Design review of the part built by this model. Coordinates are the model's own, in mm. A direction names the side the tool comes from. Give positions to 0.01 mm unless a question says otherwise; leave off trailing zeros. Loops run counter-clockwise (first coordinate to the right, second up) from the corner with the lowest first, then second, coordinate; pieces in that order, holes last. Notation, with made-up numbers: (17.5, 12.25) -> (21.5, 12.25) arc R17 cw to (21.5, 38.25) -> close; hole circle Ø10 at (87.5, 33). An arc over 180 degrees is marked (long way). Use CSV: the item, a comma, the result in double quotes. Start each with the question number.
Item 1: Clearance check with flat-ended pins moving along their axes: pin 1 (3.5 mm diameter, centred on x = 17.68, y = 17.68, fed in from +Z); pin 2 (3 mm diameter, centred on x = 19.5, y = -1.5, fed in from +Z); pin 3 (10 mm diameter, centred on x = -9.5, z = -25.5, fed in from -Y). State where each tip first meets the part, or that it passes through.
Item 2: Wall thickness on line 1 along Y through (x, z) = (0, -17); line 2 along Y through (x, z) = (0, -25); line 3 along Z through (x, y) = (-35.5, 26.5): over which ranges is each line inside the solid? List them lowest first. Write a range as from..to.
Item 3: We need section D-D (x = 31). State the section outline as (y, z) points, plus the area to 3 significant figures.
Item 4: We need section A-A (x = 0). State the section outline as (y, z) points, plus the area to 3 significant figures.
Item 5: We need section C-C (y = 30). State the section outline as (x, z) points, plus the area to 3 significant figures.
Item 6: The part is to be moulded in two halves that separate along X. For faces 1 (the face through (-20, 0, -20)), 2 (the face through (50.934, 16.04, -18.98)), 3 (the face through (-1, -11, -38.5)), say which applies: +X half, -X half, draft (parallel to the pull), parting line (faces both ways), or undercut.
Item 7: For faces 4 (the face through (-1.73, -7.81, -17.97)), 5 (the face through (20, 0, -20)), 6 (the face through (0.33, -27.52, -28.64)), list the 3-axis set-ups (+Z, -Z, +X, -X, +Y, -Y) from which the entire face can be reached by the end or side of a thin tool; tool diameter is ignored.
from build123d import *

# Parameters (mm, degrees)
SKETCH3_R           = 53.4
BOSS_EXTRUDE1_DEPTH = 38.5
SKETCH4_R           = 8
CUT_EXTRUDE1_DEPTH  = 85.766561804
SKETCH5_R           = 2
CUT_EXTRUDE2_DEPTH  = 20
BOSS_EXTRUDE3_START = 2
SKETCH6_R           = 16
SKETCH6_R_2         = 8
BOSS_EXTRUDE3_DEPTH = 2
SKETCH7_R           = 2.1
CUT_EXTRUDE3_DEPTH  = 20
SKETCH8_R           = 2.5
CUT_EXTRUDE4_DEPTH  = 20


with BuildPart() as part:
    # Sketch3 → Boss-Extrude1 (new body)
    with BuildSketch(Plane.XY):
        Circle(SKETCH3_R)
    extrude(amount=-BOSS_EXTRUDE1_DEPTH)

    # Sketch4 → Cut-Extrude1 (cut, through all)
    with BuildSketch(Plane.XY):
        Circle(SKETCH4_R)
    extrude(amount=-CUT_EXTRUDE1_DEPTH, mode=Mode.SUBTRACT)

    # Sketch5 → Cut-Extrude2 (cut)
    with BuildSketch(Plane.XY):
        with Locations((-17.67766953, 17.67766953)):
            Circle(SKETCH5_R)
        with Locations((17.67766953, 17.67766953)):
            Circle(SKETCH5_R)
        with Locations((-17.67766953, -17.67766953)):
            Circle(SKETCH5_R)
        with Locations((17.67766953, -17.67766953)):
            Circle(SKETCH5_R)
    extrude(amount=-CUT_EXTRUDE2_DEPTH, mode=Mode.SUBTRACT)

    # Sketch6 → Boss-Extrude3 (add)
    with BuildSketch(Plane.XY.offset(BOSS_EXTRUDE3_START)):
        Circle(SKETCH6_R)
        Circle(SKETCH6_R_2, mode=Mode.SUBTRACT)
    extrude(amount=-BOSS_EXTRUDE3_DEPTH)

    # Sketch7 → Cut-Extrude3 (cut)
    with BuildSketch(Plane.XY):
        with Locations((0, 20)):
            Circle(SKETCH7_R)
        with Locations((20, 0)):
            Circle(SKETCH7_R)
        with Locations((-20, 0)):
            Circle(SKETCH7_R)
        with Locations((0, -20)):
            Circle(SKETCH7_R)
    extrude(amount=-CUT_EXTRUDE3_DEPTH, mode=Mode.SUBTRACT)

    # Sketch8 → Cut-Extrude4 (cut)
    with BuildSketch(Plane(origin=(0, 0, -38.5), x_dir=(-1, 0, 0), z_dir=(0, 0, -1))):
        with Locations((0, 30)):
            Circle(SKETCH8_R)
        with Locations((30, 0)):
            Circle(SKETCH8_R)
        with Locations((0, -30)):
            Circle(SKETCH8_R)
        with Locations((-30, 0)):
            Circle(SKETCH8_R)
    extrude(amount=-CUT_EXTRUDE4_DEPTH, mode=Mode.SUBTRACT)


solid = part.part
Results found:
1,pin 1,"z = -20"
1,pin 2,"z = 0"
1,pin 3,"y = -53.21"
2,line 1,"-53.4..-22.1, -17.9..-8, 8..17.9, 22.1..53.4"
2,line 2,"-53.4..-32.5, -27.5..-8, 8..27.5, 32.5..53.4"
2,line 3,"-38.5..0"
3,outline,"(-43.48, -38.5) -> (-2.29, -38.5) -> (-2.29, -18.5) -> (2.29, -18.5) -> (2.29, -38.5) -> (43.48, -38.5) -> (43.48, 0) -> (-43.48, 0) -> close"
3,area,"3,260 mm²"
4,outline,"(-53.4, -38.5) -> (-32.5, -38.5) -> (-32.5, -18.5) -> (-27.5, -18.5) -> (-27.5, -38.5) -> (-8, -38.5) -> (-8, 2) -> (-16, 2) -> (-16, 0) -> (-17.9, 0) -> (-17.9, -20) -> (-22.1, -20) -> (-22.1, 0) -> (-53.4, 0) -> close; (8, -38.5) -> (27.5, -38.5) -> (27.5, -18.5) -> (32.5, -18.5) -> (32.5, -38.5) -> (53.4, -38.5) -> (53.4, 0) -> (22.1, 0) -> (22.1, -20) -> (17.9, -20) -> (17.9, 0) -> (16, 0) -> (16, 2) -> (8, 2) -> close"
4,area,"3,160 mm²"
5,outline,"(-44.18, -38.5) -> (-2.5, -38.5) -> (-2.5, -18.5) -> (2.5, -18.5) -> (2.5, -38.5) -> (44.18, -38.5) -> (44.18, 0) -> (-44.18, 0) -> close"
5,area,"3,300 mm²"
6,face 1,"undercut"
6,face 2,"parting line"
6,face 3,"draft"
7,face 4,"+Z, -Z"
7,face 5,"+Z"
7,face 6,"-Z"
